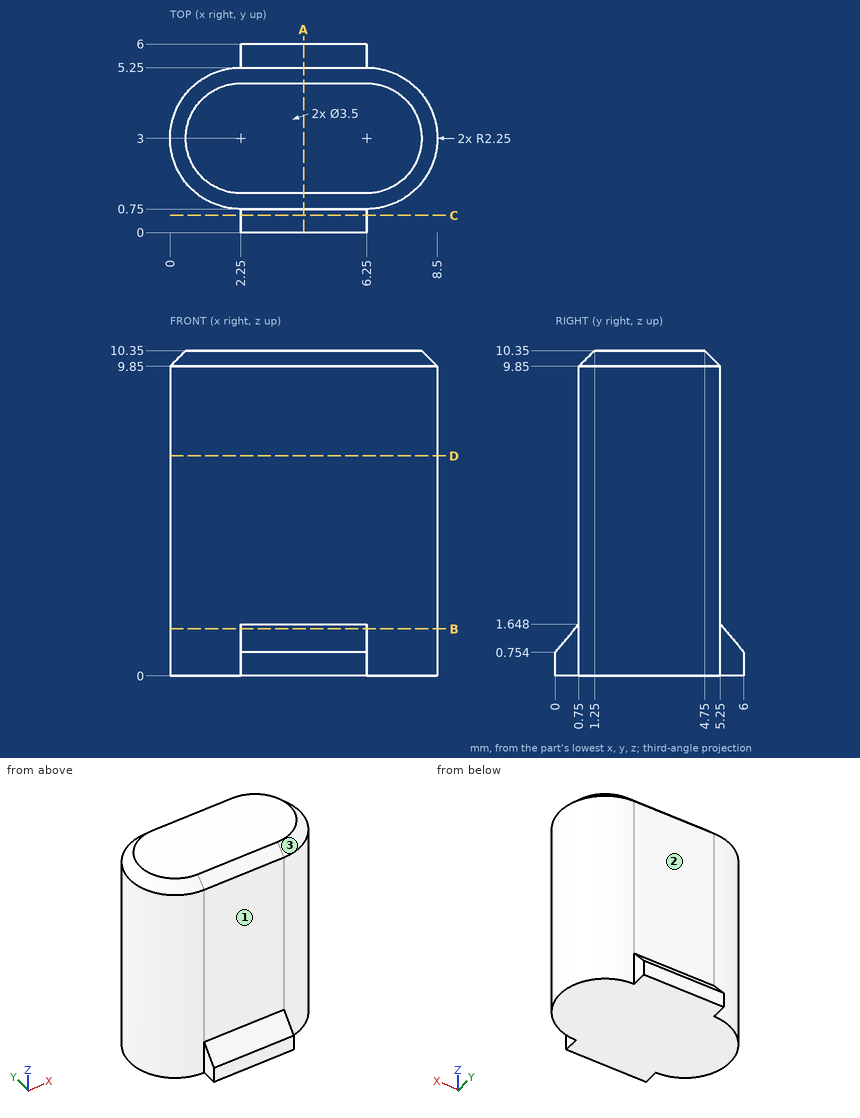
Print and shaded views of the part. All mm, measured from the part's lowest x, y and z. A direction names the side the tool comes from. Give positions to 0.01 mm unless a question says otherwise; leave off trailing zeros. Write each loop counter-clockwise with the first axis right and the second up, starting at its lowest first coordinate (ties: lowest second). Pieces come first, ordered by that corner, then holes. Notation, with made-up numbers: (45, 87.25) - (103, 87.25) arc R18 cw to (103, 94.25) - close; hole circle Ø11 at (8, 32). An arc over 180 degrees is marked (long way). One line per question, with ' | ' between items. Start each with the question number.
(1) 3-axis set-ups, long thin cutter, end or side, ignore diameter. For the marked faces 1, 2 and 3: which of +Z, -Z, +X, -X, +Y, -Y reach the whole face in a straight line?
(2) Slice it at D-D on z = 7. Write the cut outline in (x, y).
(3) Slice it at C-C on y = 0.55. Write the cut outline in (x, z).
(4) Slice it at A-A on x = 4.25. Write the cut outline in (y, z), plus the area to 3 significant figures.
(5) Pin check, flat tips, straight feed: P1, Ø0.6, axis at y = 0, z = 0.5, coming from the -X side; P2, Ø1, axis at x = 6.5, y = 3, coming from the -Z side; P3, Ø3, axis at x = 4, z = 8, coming from the +Y side; P4, Ø1.5, axis at y = 2, z = 5.5, coming from the +X side. Stop position of each tip, or through.
(6) Slice it at B-B on z = 1.5. Write the cut outline in (x, y).
(7) Wall check: line 1 along Y through (x, z) = (2.75, 4.25); line 2 along X through (y, z) = (1.7, 8.25); line 3 along Y through (x, z) = (1.5, 7.5). Give the ranges that are in metal, low to high. Write a range as from..to.
Results below:
1) face 1: +Z, +X, -X, -Y | face 2: +Z, +X, -X, +Y | face 3: +Z, +X
2) outline: (2.25, 0.75) - (6.25, 0.75) arc R2.25 ccw to (6.25, 5.25) - (2.25, 5.25) arc R2.25 ccw to start
3) outline: (2.25, 0) - (6.25, 0) - (6.25, 1.41) - (2.25, 1.41) - close
4) outline: (0, 0) - (6, 0) - (6, 0.75) - (5.25, 1.65) - (5.25, 9.85) - (4.75, 10.35) - (1.25, 10.35) - (0.75, 9.85) - (0.75, 1.65) - (0, 0.75) - close | area: 48.1 mm^2
5) P1: x = 2.25 | P2: z = 0 | P3: y = 5.25 | P4: x = 8.49
6) outline: (2.25, 0.63) - (6.25, 0.63) - (6.25, 0.75) arc R2.25 ccw to (6.25, 5.25) - (6.25, 5.37) - (2.25, 5.37) - (2.25, 5.25) arc R2.25 ccw to (2.25, 0.75) - close
7) line 1: 0.75..5.25 | line 2: 0.41..8.09 | line 3: 0.88..5.12
